Read the model definition and answer for the solid it produces. Units are mm, in the model's axes. A direction names the side the tool comes from. Coordinates: 2 decimals unless noted, no trailing zeros. Write each loop counter-clockwise with the first axis right and the second up, starting at its lowest first coordinate (ties: lowest second). Pieces come first, ordered by that corner, then holes. Notation, with made-up numbers: (88, -15.75) -> (141, -15.75) arc R23 cw to (141, -6.75) -> close; hole circle Ø6 at (-39, -10.75). An arc over 180 degrees is marked (long way). Answer in a Markdown table with one row per item. Add a question column.
Item 1: For a pull along Z with two mould halves and no side action, classify faces 1 (the face through (27, -13, 0.635)), 2 (the face through (-1, 0, 0)), 3 (the face through (-27, -1.27, -13)), 4 (the face through (1, -13, 32.385)) as +Z half, -Z half, draft (parallel to the pull), parting line (faces both ways), or undercut.
Item 2: Which of the six approach directions +Z, -Z, +X, -X, +Y, -Y give full straight-line access (tool end or side, diameter ignored) to faces 5 (the face through (-1, -25.4, 0)), 6 (the face through (-12.7, -13, -14))?
Item 3: Given pin 1 Ø7.5 at (x, z) = (-33, -9) entering from -Y, flat-ended and moving along its own axis, determine where the tip first touches the part or whether it passes through.
Item 4: Section C-C on x = 15.5 is taken. Write down the section's boundary in (y, z) (3 decimals), then the cut area to 3 significant figures.
Item 5: Section A-A on y = -22.5 is taken. Count the separate pieces of the cut face and the enclosed holes in it, then the cut area to 3 significant figures.
Item 6: Section B-B on z = 15.5 is taken. Write down the section's boundary in (x, y).
Item 7: Straight lines are drawn through the part: line 1 (Z direction, x = -32.5, y = -24) (3 decimals); line 2 (X direction, y = -4.75, z = -9); line 3 (Y direction, x = -14.5, z = 15.5). For each, find the intervals that lie inside material, in ascending order. Write a range as from..to.
```python
from build123d import *

# Parameters (mm, degrees)
F0_W     = 25.4
F0_H     = 25.4
F1_DEPTH = 25.4
F2_W     = 91.44
F2_H     = 64.77
F3_DEPTH = 1.27
F4_R     = 5.08


with BuildPart() as f1:
    # F0 (on Front) → F1 (new body)
    with BuildSketch(Plane.XZ):
        Polygon((-45.72, -32.385), (45.72, -32.385), (45.72, 32.385), (-38.428448, 32.385), (-45.72, 32.385), (-45.72, 27.392585), align=None)
        Polygon((-39.37, -0.635), (-36.457758, -0.635), (-13.97, -0.635), (-13.97, -26.035), (-39.37, -26.035), align=None, mode=Mode.SUBTRACT)
        with Locations((0, -13.335)):
            Rectangle(F0_W, F0_H, mode=Mode.SUBTRACT)
        with Locations((26.67, -13.335)):
            Rectangle(F0_W, F0_H, mode=Mode.SUBTRACT)
        Polygon((-39.37, 26.035), (-38.428448, 26.035), (-13.97, 26.035), (-13.97, 13.335), (-13.97, 0.635), (-36.457758, 0.635), (-39.37, 0.635), align=None, mode=Mode.SUBTRACT)
        Polygon((-12.7, 0.635), (-12.7, 13.335), (-12.7, 26.035), (12.7, 26.035), (12.7, 15.568449), (12.7, 0.635), align=None, mode=Mode.SUBTRACT)
        Polygon((13.97, 0.635), (13.97, 15.568449), (13.97, 26.035), (39.37, 26.035), (39.37, 0.635), align=None, mode=Mode.SUBTRACT)
    extrude(amount=F1_DEPTH)

    # F2 (on Front) → F3 (join)
    with BuildSketch(Plane.XZ):
        Rectangle(F2_W, F2_H)
    extrude(amount=F3_DEPTH)

    # F4
    f4_edges = [f1.edges().sort_by_distance(p)[0] for p in [
        (-45.72, -12.7, 32.385),
        (45.72, -12.7, 32.385),
        (-45.72, -12.7, -32.385),
        (45.72, -12.7, -32.385),
    ]]
    fillet(f4_edges, radius=F4_R)


solid = f1.part
```
Results below:
| question | item | result |
|---|---|---|
| 1 | face 1 | undercut |
| 1 | face 2 | draft |
| 1 | face 3 | undercut |
| 1 | face 4 | +Z half |
| 2 | face 5 | +Z, -Z, +X, -X, -Y |
| 2 | face 6 | -Y |
| 3 | pin 1 | stops at y = -1.27 |
| 4 | outline | (-25.4, -32.385) -> (0, -32.385) -> (0, 32.385) -> (-25.4, 32.385) -> (-25.4, 26.035) -> (-1.27, 26.035) -> (-1.27, 0.635) -> (-25.4, 0.635) -> (-25.4, -0.635) -> (-1.27, -0.635) -> (-1.27, -26.035) -> (-25.4, -26.035) -> close |
| 4 | area | 419 mm2 |
| 5 | separate pieces | 1 |
| 5 | enclosed holes | 6 |
| 5 | area | 2,030 mm2 |
| 6 | outline | (-45.72, -25.4) -> (-39.37, -25.4) -> (-39.37, -1.27) -> (-13.97, -1.27) -> (-13.97, -25.4) -> (-12.7, -25.4) -> (-12.7, -1.27) -> (12.7, -1.27) -> (12.7, -25.4) -> (13.97, -25.4) -> (13.97, -1.27) -> (39.37, -1.27) -> (39.37, -25.4) -> (45.72, -25.4) -> (45.72, 0) -> (-45.72, 0) -> close |
| 7 | line 1 | z = -32.385..-26.035, -0.635..0.635, 26.035..32.385 |
| 7 | line 2 | x = -45.72..-39.37, -13.97..-12.7, 12.7..13.97, 39.37..45.72 |
| 7 | line 3 | y = -1.27..0 |
